```python
from build123d import *

# Parameters (mm, degrees)
SKETCH_1_R      = 6.25
SKETCH_1_R_2    = 4.5
EXTRUDE_1_DEPTH = 8
EXTRUDE_2_DEPTH = 4.5


with BuildPart() as part:
    # 草图1 → 凸台-拉伸1 (new body)
    with BuildSketch(Plane(origin=(0, 0, 0), x_dir=(1, 0, 0), z_dir=(0, 1, 0))):
        with Locations(Location((0, 0, 0), (0, 0, 270))):
            Circle(SKETCH_1_R)
        with Locations(Location((0, 0, 0), (0, 0, 270))):
            Circle(SKETCH_1_R_2, mode=Mode.SUBTRACT)
    extrude(amount=EXTRUDE_1_DEPTH)

    # 草图2 → 凸台-拉伸2 (add)
    with BuildSketch(Plane(origin=(0, 8, 0), x_dir=(1, 0, 0), z_dir=(0, 1, 0))):
        Polygon((4.25, 7.361215932), (-4.25, 7.361215932), (-8.5, 0), (-4.25, -7.361215932), (4.25, -7.361215932), (8.5, 0), align=None)
    extrude(amount=EXTRUDE_2_DEPTH)

    # 草图3 → 旋转1 (revolve)
    with BuildSketch(Plane.XY, mode=Mode.PRIVATE) as revolve_1_sk:
        with BuildLine():
            ThreePointArc((6, 14.1), (6.729436981, 13.443398113), (7, 12.5))
            Line((7, 12.5), (0, 12.5))
            Line((0, 12.5), (0, 14))
            Line((0, 14), (6, 14))
            Line((6, 14), (6, 14.1))
        make_face()
    revolve(revolve_1_sk.sketch.rotate(Axis((0, -20.81110882, 0), (0, 1, 0)), 90), axis=Axis((0, -20.81110882, 0), (0, 1, 0)))


solid = part.part
```
Build history of the part. All positions in model axes, mm. A direction names the side the tool comes from. Round coordinates to 2 decimals unless told otherwise and drop trailing zeros. Loops run counter-clockwise (first coordinate to the right, second up) from the corner with the lowest first, then second, coordinate; pieces in that order, holes last. Notation, with made-up numbers: M 43,10.25 L 87,10.25 A11 cw 87,20.25 Z; hole C -9,-4 d3. An arc over 180 degrees is marked long. Answer as CSV lines item,"result".
1. 3-axis set-ups, long thin cutter, end or side, ignore diameter. For faces 1 (the flat face through (7, 12.5, -2)), 2 (the flat face through (0, 10, -7.361)), 3 (the flat face through (0, 8, 0)): which of +Z, -Z, +X, -X, +Y, -Y reach the whole face in a straight line?
Resolved:
face 1,"+Y"
face 2,"-Z, +X, -X, +Y, -Y"
face 3,"-Y"
2. Wall check: probe 1 along X at (y, z) = (2.5, 0); probe 2 along Y at (x, z) = (1.25, 2.5); probe 3 along X at (y, z) = (3.5, -3). Give the ranges that are in metal, low to high. Write a range as [from, to].
Resolved:
probe 1,"x = [-6.25, -4.5], [4.5, 6.25]"
probe 2,"y = [8, 14]"
probe 3,"x = [-5.48, -3.35], [3.35, 5.48]"
3. Cut at B-B on y = 3.5. Write the cut outline in (x, z).
Resolved:
outline,"C 0,0 d12.5; hole C 0,0 d9"
4. Flat gauge pins, fed straight in: P1, Ø1.5, axis at x = -0.5, z = -2.5, coming from the +Y side; P2, Ø8, axis at y = 11, z = -1.5, coming from the -X side; P3, Ø3, axis at y = 12.5, z = -4.5, coming from the +X side; P4, Ø2, axis at x = -3.5, y = 4.5, coming from the +Z side. Where does each tip first touch, or does it go through?
Resolved:
P1,"stops at y = 14"
P2,"stops at x = -8.5"
P3,"stops at x = 6.77"
P4,"stops at z = 5.73"
5. Two-plate mould, pull along Z, no slides. Class faces 4 (the flat face through (-6.405, 10.218, 3.629)), 5 (the flat face through (0, 14, 0)), 6 (the flat face through (6.405, 10.218, -3.629)): released by +Z, released by -Z, zero draft, split by the parting line, or undercut.
Resolved:
face 4,"released by +Z"
face 5,"undercut"
face 6,"released by -Z"
6. Cut at A-A on x = 0. Write the cut outline in (y, z).
Resolved:
outline,"M 0,-6.25 L 8,-6.25 L 8,-7.36 L 12.5,-7.36 L 12.5,-7 A1.78 ccw 14.1,-6 L 14,-6 L 14,6 L 14.1,6 A1.78 ccw 12.5,7 L 12.5,7.36 L 8,7.36 L 8,6.25 L 0,6.25 L 0,4.5 L 8,4.5 L 8,-4.5 L 0,-4.5 Z"
7. Cut at C-C on y = 8.25. Write the cut outline in (x, z).
Resolved:
outline,"M -8.5,0 L -4.25,-7.36 L 4.25,-7.36 L 8.5,0 L 4.25,7.36 L -4.25,7.36 Z"
